Source: three-view drawing plus pictorial views. Frame: mm from the lowest corner of the part. Coordinates: 2 decimals unless noted, no trailing zeros. Write each loop counter-clockwise with the first axis right and the second up, starting at its lowest first coordinate (ties: lowest second). Pieces come first, ordered by that corner, then holes. Notation, with made-up numbers: (59, -39.75) - (68, -39.75) arc R23 cw to (68, -8.75) - close; hole circle Ø4 at (-8, -27.75). An arc over 180 degrees is marked (long way). Put each result on its own line as item: value. Start each with the question number.
1. Pin query (flat end, axial travel): pin 1 (8 mm diameter, centred on y = 93.5, z = 14, fed in from +X); pin 2 (2 mm diameter, centred on x = 264.5, z = 12.5, fed in from -Y). Return the tip coordinate at first contact, or that it passes through.
2. Cut plane A-A, the plane z = 11.75. Return loops of the section in (x, y), and give its area (3 significant figures).
3. Cut plane B-B, the plane x = 351. Return loops of the section in (y, z), and give its area (3 significant figures).
4. Line query: line 1 (Y direction, x = 372.5, z = 16); line 2 (X direction, y = 59, z = 11.75); line 3 (X direction, y = 127.5, z = 8). Output: solid intervals per line, ascending.
5. Cut plane C-C, the plane y = 57. Return loops of the section in (x, z).
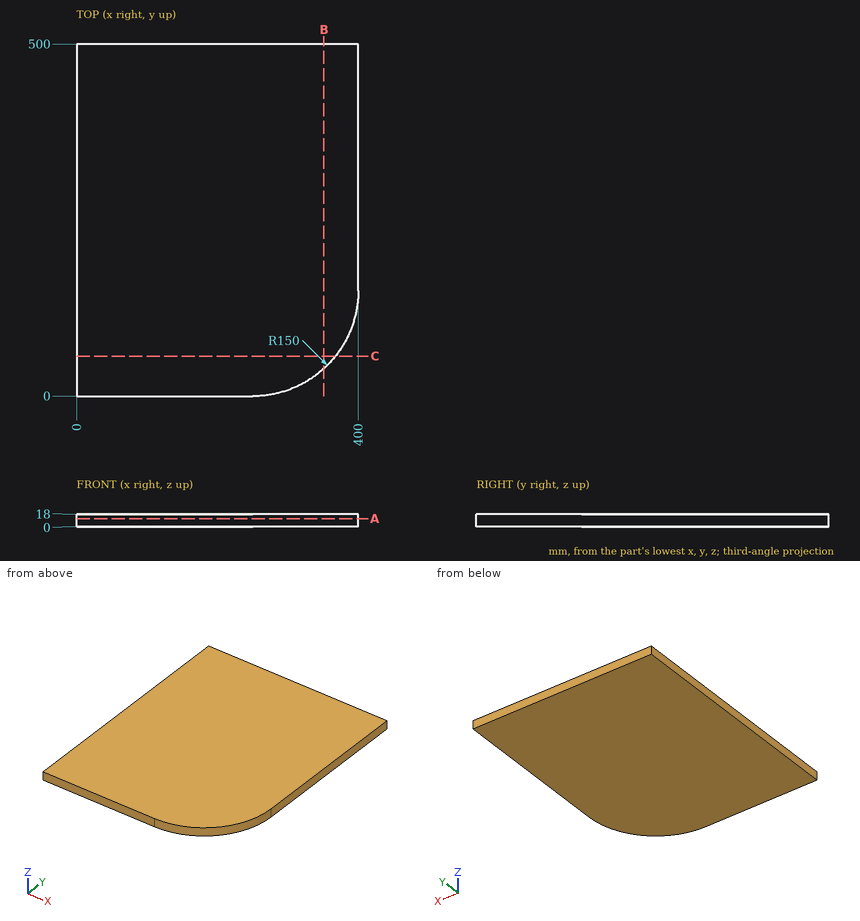
Report:
1. pin 1: stops at x = 390.51
1. pin 2: stops at y = 0.61
2. outline: (0, 0) - (250, 0) arc R150 ccw to (400, 150) - (400, 500) - (0, 500) - close
2. area: 195,000 mm^2
3. outline: (39.1, 0) - (500, 0) - (500, 18) - (39.1, 18) - close
3. area: 8,300 mm^2
4. line 1: y = 63.43 to 500
4. line 2: x = 0 to 369.24
4. line 3: x = 0 to 398.3
5. outline: (0, 0) - (367.69, 0) - (367.69, 18) - (0, 18) - close
